Here's how the part is built. I have some questions about the finished solid (model axes, mm). A direction names the side the tool comes from. Give positions to 0.01 mm unless a question says otherwise; leave off trailing zeros. Write each loop counter-clockwise with the first axis right and the second up, starting at its lowest first coordinate (ties: lowest second). Pieces come first, ordered by that corner, then holes. Notation, with made-up numbers: (25, 85) -> (69, 85) arc R3 cw to (69, 89) -> close; hole circle Ø11 at (18, 15). An arc over 180 degrees is marked (long way). Use one line per item in the form item = value.
```python
from build123d import *

# Parameters (mm, degrees)
F1_DEPTH = 19.05
F2_DEPTH = 25.4
F3_T     = -5.08


# Not quite as in the source:
# - a feature names something its author has since deleted; it is built from what else it names


with BuildPart() as f1:
    # F0 (on Front) → F1 (new body)
    with BuildSketch(Plane.XZ):
        with BuildLine():
            ThreePointArc((12.7, 21.9970452561), (-21.4428837855, 13.6147983812), (-14.5054559874, -20.8507013455))
            ThreePointArc((-14.5054559874, -20.8507013455), (-1.0693193728, -25.3774812793), (12.7, -21.9970452561))
            ThreePointArc((12.7, -21.9970452561), (0, 0), (12.7, 21.9970452561))
        make_face()
    extrude(amount=F1_DEPTH)

    # F0 (on Front) → F2 (join)
    with BuildSketch(Plane.XZ):
        with BuildLine():
            ThreePointArc((12.7, 21.9970452561), (-21.4428837855, 13.6147983812), (-14.5054559874, -20.8507013455))
            ThreePointArc((-14.5054559874, -20.8507013455), (-1.0693193728, -25.3774812793), (12.7, -21.9970452561))
            ThreePointArc((12.7, -21.9970452561), (0, 0), (12.7, 21.9970452561))
        make_face()
        with BuildLine():
            ThreePointArc((12.7, -21.9970452561), (-1.0693193728, -25.3774812793), (-14.5054559874, -20.8507013455))
            Line((-14.5054559874, -20.8507013455), (12.7, -39.7770452561))
            Line((12.7, -39.7770452561), (12.7, -21.9970452561))
        make_face()
        with BuildLine():
            ThreePointArc((12.7, 21.9970452561), (0, 0), (12.7, -21.9970452561))
            ThreePointArc((12.7, -21.9970452561), (21.9970452561, -12.7), (25.4, 0))
            ThreePointArc((25.4, 0), (21.9970452561, 12.7), (12.7, 21.9970452561))
        make_face()
        with BuildLine():
            ThreePointArc((25.4, 0), (21.9970452561, -12.7), (12.7, -21.9970452561))
            ThreePointArc((12.7, -21.9970452561), (26.4693193728, -25.3774812793), (39.9054559874, -20.8507013455))
            ThreePointArc((39.9054559874, -20.8507013455), (47.9122031583, -11.762682898), (50.8, 0))
            ThreePointArc((50.8, 0), (38.1, 21.9970452561), (12.7, 21.9970452561))
            ThreePointArc((12.7, 21.9970452561), (21.9970452561, 12.7), (25.4, 0))
        make_face()
        with BuildLine():
            ThreePointArc((39.9054559874, -20.8507013455), (26.4693193728, -25.3774812793), (12.7, -21.9970452561))
            Line((12.7, -21.9970452561), (12.7, -39.7770452561))
            Line((12.7, -39.7770452561), (39.9054559874, -20.8507013455))
        make_face()
    extrude(amount=F2_DEPTH)

    # F3
    f3_openings = [f1.faces().sort_by_distance(p)[0] for p in [
        (12.7, -25.4, -2.767667),
    ]]
    offset(amount=F3_T, openings=f3_openings, kind=Kind.INTERSECTION)


solid = f1.part
```
Q1. I want a section at C-C, the plane z = -2. Write out the boundary of the cut face in (x, y), and give its area (3 significant figures).
Result set:
outline = (-25.32, -25.4) -> (-20.22, -25.4) -> (-20.22, -5.08) -> (45.62, -5.08) -> (45.62, -25.4) -> (50.72, -25.4) -> (50.72, 0) -> (-25.32, 0) -> close
area = 594 mm2
Q2. If we mould it in two halves opening along X, with no side actions, what happens to faces 1 (the face through (-1.093, -12.522, -30.181)), 2 (the face through (26.11, -12.52, -30.45)), 3 (the face through (12, -5.08, 0))? For each: +X half, -X half, draft (parallel to the pull), parting line (faces both ways), or undercut.
Result set:
face_1 = -X half
face_2 = +X half
face_3 = undercut
Q3. Will these pins go through, and if not, where does the flat tip stop? pin 1 Ø6 at (x, y) = (26, -8) entering from -Z; pin 2 Ø3 at (x, y) = (-16.5, -4.5) entering from -Z; pin 3 Ø1.5 at (x, y) = (38, -19) entering from -Z.
Result set:
pin_1 = -32.61
pin_2 = -20.5
pin_3 = -22.7
Q4. Which directions (+Z, -Z, +X, -X, +Y, -Y) give clear straight access to the entire face, cutting with the end or side of a thin tool? Please do faces 4 (the face through (-21.147, -12.522, 14.071)), 5 (the face through (0.38, -15.1, -25.02)).
Result set:
face_4 = +Y, -Y
face_5 = -Y
Q5. I want a section at B-B, the plane x = 0. Write out the boundary of the cut face in (y, z).
Result set:
outline = (-25.4, -30.94) -> (0, -30.94) -> (0, 25.4) -> (-25.4, 25.4) -> (-25.4, 20.32) -> (-5.08, 20.32) -> (-5.08, -24.75) -> (-25.4, -24.75) -> close
Q6. If I drill on line 1 along Y through (x, z) = (24.5, -22); line 2 along Z through (x, y) = (7, -10.5); line 3 along Z through (x, y) = (-7.5, -14.75), over which ranges is the centre line in solid material (lowest first)? Write a range as from..to.
Result set:
line_1 = -5.08..0
line_2 = -35.81..-29.62, 19.08..24.42
line_3 = -25.72..-19.54, 18.89..24.27
Q7. I want a section at A-A, the plane y = -16.75. Write out the boundary of the cut face in (x, z).
Result set:
outline = (-14.51, -20.85) -> (12.7, -39.78) -> (39.91, -20.85) arc R25.4 ccw to (12.7, 22) arc R25.4 ccw to start; hole (-11.6, -16.68) -> (12.7, -33.59) -> (37, -16.68) arc R20.32 ccw (long way) to (12.7, 15.86) arc R20.32 ccw (long way) to start
